from build123d import *

# Parameters (mm, degrees)
BOSS_EXTRUDE1_DEPTH = 6
M4_TAPPED_HOLE5_D   = 3.3
LPATTERN3_COUNT     = 2
LPATTERN3_PITCH     = 75
LPATTERN4_COUNT     = 2
LPATTERN4_PITCH     = 20
SKETCH15_R          = 3.75
CUT_EXTRUDE1_DEPTH  = 4
SKETCH16_R          = 3.75
CUT_EXTRUDE3_DEPTH  = 4


with BuildPart() as part:
    # Sketch1 → Boss-Extrude1 (new body)
    with BuildSketch(Plane(origin=(0, 0, 0), x_dir=(1, 0, 0), z_dir=(0, 1, 0))):
        with BuildLine():
            Line((-40, 15), (40, 15))
            ThreePointArc((40, 15), (55, 0), (40, -15))
            Line((40, -15), (-40, -15))
            ThreePointArc((-40, -15), (-55, 0), (-40, 15))
        make_face()
    extrude(amount=BOSS_EXTRUDE1_DEPTH)

    # Sketch4 → M4 Tapped Hole3 (revolve, cut)
    with BuildSketch(Plane(origin=(37.5, 6, 0), x_dir=(0, 0, 1), z_dir=(1, 0, 0))):
        Polygon((0, 0), (0, 12.491420021), (1.65, 11.5), (1.65, 0), align=None)
    m4_tapped_hole3 = revolve(axis=Axis((37.5, 12.35, 0), (0, -1, 0)), mode=Mode.SUBTRACT)

    # M4 Tapped Hole5 (through all)
    with Locations(Plane(origin=(10, 6, 0), x_dir=(0, 0, 1), z_dir=(0, 1, 0))):
        with Locations((0, 0)):
            m4_tapped_hole5 = Hole(M4_TAPPED_HOLE5_D / 2)

    # LPattern3: M4 Tapped Hole3 ×2
    with Locations(*[(-i * LPATTERN3_PITCH, 0, 0) for i in range(1, LPATTERN3_COUNT)]):
        add(m4_tapped_hole3, mode=Mode.SUBTRACT)

    # LPattern4: M4 Tapped Hole5 ×2
    with Locations(*[(-i * LPATTERN4_PITCH, 0, 0) for i in range(1, LPATTERN4_COUNT)]):
        add(m4_tapped_hole5, mode=Mode.SUBTRACT)

    # Sketch15 → Cut-Extrude1 (cut)
    with BuildSketch(Plane(origin=(0, 6, 0), x_dir=(1, 0, 0), z_dir=(0, 1, 0))):
        with Locations(Location((37.5, 0, 0), (0, 0, 270))):
            Circle(SKETCH15_R)
        with Locations(Location((-37.5, 0, 0), (0, 0, 270))):
            Circle(SKETCH15_R)
    extrude(amount=-CUT_EXTRUDE1_DEPTH, mode=Mode.SUBTRACT)

    # Sketch16 → Cut-Extrude3 (cut)
    with BuildSketch(Plane.XZ):
        with Locations(Location((-10, 0, 0), (0, 0, 270))):
            Circle(SKETCH16_R)
        with Locations(Location((10, 0, 0), (0, 0, 270))):
            Circle(SKETCH16_R)
    extrude(amount=-CUT_EXTRUDE3_DEPTH, mode=Mode.SUBTRACT)


solid = part.part
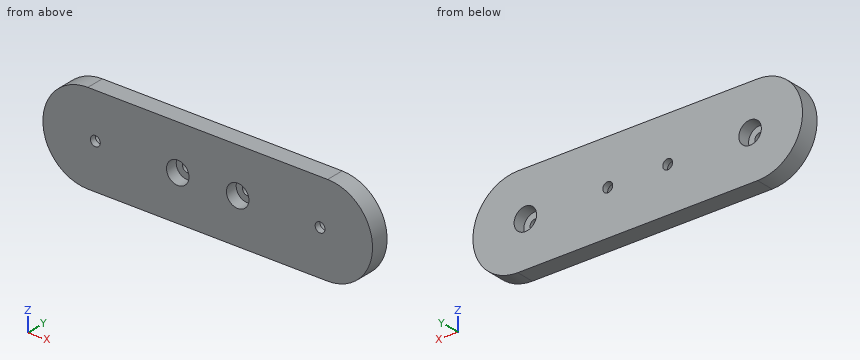
Input: part model. Units: mm. Frame: model coordinates. Coordinates: 2 decimals unless noted, no trailing zeros. Loops run counter-clockwise (first coordinate to the right, second up) from the corner with the lowest first, then second, coordinate; pieces in that order, holes last. Notation, with made-up numbers: (-29.5, 71) - (-2.5, 71) arc R27 cw to (-2.5, 102) - close; hole circle Ø6 at (50.25, -36). An arc over 180 degrees is marked (long way). Answer in a Markdown table with one row per item. Add a question column.
Item 1: Section query A-A on y = 4.9. Return the cut outline in (x, z), then the cut area to 3 significant figures.
Item 2: Contact query for flat-ended pins moving along their axis: P1, Ø4.5, axis at x = 10, z = 0, coming from the -Y side; P2, Ø3, axis at x = 37.5, z = 0, coming from the +Y side; P3, Ø3, axis at y = 2, z = 3, coming from the -X side. Output: stop coordinate, or through.
Item 3: Line query: line 1 along X through (y, z) = (1.55, 0); line 2 along X through (y, z) = (4.6, 0); line 3 along Y through (x, z) = (-36, -3). Output: solid intervals per line, ascending. Write a range as [from, to].
Item 4: Section query B-B on x = 10. Return the cut outline in (y, z), then the cut area to 3 significant figures.
Item 5: Section query D-D on z = 11. Return the cut outline in (x, y), then the cut area to 3 significant figures.
Item 6: Section query C-C on z = 0. State how many separate pieces and enclosed holes the cut face has, then the cut area to 3 significant figures.
Recorded:
| question | item | result |
|---|---|---|
| 1 | outline | (-40, -15) - (40, -15) arc R15 ccw to (40, 15) - (-40, 15) arc R15 ccw to start; hole circle Ø7.5 at (-37.5, 0); hole circle Ø3.3 at (-10, 0); hole circle Ø3.3 at (10, 0); hole circle Ø7.5 at (37.5, 0) |
| 1 | area | 3,000 mm^2 |
| 2 | P1 | y = 4 |
| 2 | P2 | through |
| 2 | P3 | x = -54.92 |
| 3 | line 1 | [-55, -39.15], [-35.85, -13.75], [-6.25, 6.25], [13.75, 35.85], [39.15, 55] |
| 3 | line 2 | [-55, -41.25], [-33.75, -11.65], [-8.35, 8.35], [11.65, 33.75], [41.25, 55] |
| 3 | line 3 | [0, 2] |
| 4 | outline | (0, -15) - (6, -15) - (6, -1.65) - (4, -1.65) - (4, -3.75) - (0, -3.75) - close; (0, 3.75) - (4, 3.75) - (4, 1.65) - (6, 1.65) - (6, 15) - (0, 15) - close |
| 4 | area | 143 mm^2 |
| 5 | outline | (-50.2, 0) - (50.2, 0) - (50.2, 6) - (-50.2, 6) - close |
| 5 | area | 602 mm^2 |
| 6 | separate pieces | 5 |
| 6 | enclosed holes | 0 |
| 6 | area | 514 mm^2 |
